Autodesk Inventor part; units mm, degrees
ref_plane "YZ Plane" through (0, 0, 0) normal (1, 0, 0) x (0, 1, 0)
ref_plane "XZ Plane" through (0, 0, 0) normal (0, 1, 0) x (-1, 0, 0)
ref_plane "XY Plane" through (0, 0, 0) normal (0, 0, 1) x (1, 0, 0)
sketch "Sketch2" plane through (0, 0, 0) normal (0, 0, 1) x (1, 0, 0)
  line L0 (7, -3) -> (7, 3)
  line L1 (7, -3) -> (-7, -3)
  line L2 (-7, -3) -> (-7, 3)
  line L3 (6, 3) -> (6, 3.8)
  line L4 (6.2, 4) -> (6.8, 4)
  line L5 (7, 3.8) -> (7, 3)
  line L6 (-6, 3) -> (-6, 3.8)
  line L7 (-6.2, 4) -> (-6.8, 4)
  line L8 (-7, 3.8) -> (-7, 3)
  line L9 (-6, 3) -> (6, 3)
  line L10 (7, 3) -> (7.3028, 3)
  line L11 (-7, 3) -> (-7.3058, 3)
  arc A0 (-6, 3.8) -> (-6.2, 4) centre (-6.2, 3.8) ccw
  arc A1 (-6.8, 4) -> (-7, 3.8) centre (-6.8, 3.8) ccw
  arc A2 (6.2, 4) -> (6, 3.8) centre (6.2, 3.8) ccw
  arc A3 (7, 3.8) -> (6.8, 4) centre (6.8, 3.8) ccw
  point P0 (0, 0)
  dimension "d5" = 14
  dimension "d6" = 6
extrude "Extrusion1" add sketch "Sketch2" along normal blind 1
sketch "Sketch3" plane through (-6.8, 4, 0) normal (0, 1, 0) x (1, 0, 0)
  circle A0 centre (0.3, -0.5) radius 0.3
  point P0 (6.8, 0)
  dimension "d9" = 0.6
sketch "Sketch4" plane through (6.2, 4, 0) normal (0, 1, 0) x (1, 0, 0)
  circle A0 centre (0.3, -0.5) radius 0.3
  point P0 (-6.2, 0)
  dimension "d10" = 0.6
extrude "Extrusion2" add sketch "Sketch4" along normal blind 24
extrude "Extrusion3" add sketch "Sketch3" along normal blind 24
equation "\"BendRadius\" = Thickness"
equation "\"BendReliefWidth\" = Thickness"
equation "\"BendReliefDepth\" = 0.5 * Thickness"
equation "\"CornerReliefSize\" = 4 * Thickness"
equation "\"MinimumRemnant\" = 2 * Thickness"
equation "\"TransitionRadius\" = BendRadius"
equation "\"JacobiRadiusSize\" = BendRadius"
equation "\"GapSize\" = Thickness"
properties part number "K71-6"
Design review of the part built by this model. Coordinates are the model's own, in mm. Give positions to 0.01 mm unless a question says otherwise; leave off trailing zeros. Loops run counter-clockwise (first coordinate to the right, second up) from the corner with the lowest first, then second, coordinate; pieces in that order, holes last. Notation, with made-up numbers: M -8.5,-1 L 46.5,-1 A23 ccw 46.5,7 Z; hole C 47.25,71 d7. An arc over 180 degrees is marked long. Return JSON: item names as keys, results as strings. Group by question number.
Item 1: For probe 1 along X at (y, z) = (3.5, 0.35); probe 2 along X at (y, z) = (11.5, 0.55); probe 3 along Y at (x, z) = (4.75, 0.3), list the stretches that pass through material, from the lowest coordinate up.
Item 2: We need section A-A (x = -6.5). Give the boundary of the cut face in (y, z), and give its area (3 significant figures).
Item 3: We need section B-B (y = 21). Give the boundary of the cut face in (x, z).
Item 4: Mouldability with a two-part tool opening along X and no side actions: class faces 1 (the flat face through (0, 1, 1)), 2 (the flat face through (-7, 0.4, 0.5)), 3 (the flat face through (-0.1, 3, 0.5)) as released by +X, released by -X, zero draft, split by the parting line, or undercut.
Item 5: Insertion check: pin 1 Ø5 at (x, y) = (-5, 14.5) entering from -Z. The pin has a flat end and moves straight along its axis. Give the tip position at first contact, or say it passes through.
Item 6: We need section C-C (x = -4). Give the boundary of the cut face in (y, z).
Output:
{
 "1": {"probe 1": "x = -7 to -6, 6 to 7", "probe 2": "x = -6.8 to -6.2, 6.2 to 6.8", "probe 3": "y = -3 to 3"},
 "2": {"outline": "M -3,0 L 4,0 L 4,0.2 L 28,0.2 L 28,0.8 L 4,0.8 L 4,1 L -3,1 Z", "area": "21.4 mm^2"},
 "3": {"outline": "C -6.5,0.5 d0.6; C 6.5,0.5 d0.6"},
 "4": {"face 1": "zero draft", "face 2": "released by -X", "face 3": "undercut"},
 "5": {"pin 1": "stops at z = 0.2"},
 "6": {"outline": "M -3,0 L 3,0 L 3,1 L -3,1 Z"}
}
